Here's how the part is built. I have some questions about the finished solid (model axes, mm). Coordinates: 2 decimals unless noted, no trailing zeros. Write each loop counter-clockwise with the first axis right and the second up, starting at its lowest first coordinate (ties: lowest second). Pieces come first, ordered by that corner, then holes. Notation, with made-up numbers: (89, 62.25) -> (109, 62.25) arc R14 ccw to (109, 69.25) -> close; hole circle Ø10 at (62.25, -13). An arc over 180 degrees is marked (long way). Put each result on its own line as item: value. Start each with the question number.
Item 1: I want a section at D-D, the plane x = -8.5. List the corners of the cut face in (y, z) for me.
Item 2: For pin 1 (2 mm diameter, centred on x = -27, z = 4, fed in from +Y); pin 2 (3 mm diameter, centred on x = -3.5, y = 3.5, fed in from +Z); pin 3 (1 mm diameter, centred on x = -24, z = 2, fed in from -Y), each with a flat end and sliding along its axis, tell me the tip position at first contact or that it passes through.
Item 3: I want a section at A-A, the plane z = 1.4. List the corners of the cut face in (x, y) for me.
Item 4: I want a section at B-B, the plane y = 19. List the corners of the cut face in (x, z) for me, then the cut area to 3 significant figures.
Item 5: I need wall thicknesses on line 1 (Y direction, x = -3.5, z = 1.5); line 2 (X direction, y = 3.75, z = 4.55); line 3 (Y direction, x = -1.5, z = 2). Which ranges of each line are inside material? Lowest first, please. Write a range as [from, to].
Item 6: If we mould it in two halves opening along X, with no side actions, what happens to faces 1 (the face through (-17, 11, 5)), 2 (the face through (-5.003, 11.33, 2.465)), 3 (the face through (-16.83, 2.84, 2.46))? For each: released by +X, released by -X, zero draft, split by the parting line, or undercut.
Item 7: I want a section at C-C, the plane x = -30.5. List the corners of the cut face in (y, z) for me, then the cut area to 3 significant figures.
from build123d import *

# Parameters (mm, degrees)
ESQUISSE1_W        = 34
ESQUISSE1_H        = 22.5
ESQUISSE1_R        = 1
BOSS_EXTRU_1_DEPTH = 5
CUT_EXTRUDE1_DEPTH = 10


with BuildPart() as part:
    # Esquisse1 → Boss.-Extru.1 (new body)
    with BuildSketch(Plane.XY):
        with Locations((-17, 11.25)):
            Rectangle(ESQUISSE1_W, ESQUISSE1_H)
        with Locations((-30.5, 19)):
            Circle(ESQUISSE1_R, mode=Mode.SUBTRACT)
        with Locations((-3.5, 19)):
            Circle(ESQUISSE1_R, mode=Mode.SUBTRACT)
        with Locations((-3.5, 3.5)):
            Circle(ESQUISSE1_R, mode=Mode.SUBTRACT)
        with Locations((-30.5, 3.5)):
            Circle(ESQUISSE1_R, mode=Mode.SUBTRACT)
    extrude(amount=BOSS_EXTRU_1_DEPTH)

    # Sketch1 → Cut-Extrude1 (cut)
    with BuildSketch(Plane(origin=(0, 0, 0), x_dir=(-1, 0, 0), z_dir=(0, 0, -1))):
        Polygon((35.959040793, 25.036749556), (37.525504355, -3.285522646), (-6.460348748, -5.71831602), (-8.02681231, 22.603956182), align=None)
        with BuildLine():
            ThreePointArc((31.940553528, 15.810202901), (33.696545455, 20.425516451), (29.089552239, 22.203222926))
            ThreePointArc((29.089552239, 22.203222926), (17, 19.659419434), (4.910447761, 22.203222926))
            ThreePointArc((4.910447761, 22.203222926), (0.303454545, 20.425516451), (2.059446472, 15.810202901))
            ThreePointArc((2.059446472, 15.810202901), (5.003675676, 11.25), (2.059446472, 6.689797099))
            ThreePointArc((2.059446472, 6.689797099), (0.303454545, 2.074483549), (4.910447761, 0.296777074))
            ThreePointArc((4.910447761, 0.296777074), (17, 2.840580566), (29.089552239, 0.296777074))
            ThreePointArc((29.089552239, 0.296777074), (33.696545455, 2.074483549), (31.940553528, 6.689797099))
            ThreePointArc((31.940553528, 6.689797099), (28.996324324, 11.25), (31.940553528, 15.810202901))
        make_face(mode=Mode.SUBTRACT)
    extrude(amount=-CUT_EXTRUDE1_DEPTH, mode=Mode.SUBTRACT)


solid = part.part
Calculated:
1. outline: (1.61, 0) -> (20.89, 0) -> (20.89, 5) -> (1.61, 5) -> close
2. pin 1: stops at y = 21.75
2. pin 2: stops at z = 5
2. pin 3: stops at y = 1.89
3. outline: (-31.94, 6.69) arc R3.5 ccw to (-29.09, 0.3) arc R30 cw to (-4.91, 0.3) arc R3.5 ccw to (-2.06, 6.69) arc R5 cw to (-2.06, 15.81) arc R3.5 ccw to (-4.91, 22.2) arc R30 cw to (-29.09, 22.2) arc R3.5 ccw to (-31.94, 15.81) arc R5 cw to start; hole circle Ø2 at (-30.5, 3.5); hole circle Ø2 at (-30.5, 19); hole circle Ø2 at (-3.5, 3.5); hole circle Ø2 at (-3.5, 19)
4. outline: (-34, 0) -> (-31.5, 0) -> (-31.5, 5) -> (-34, 5) -> close; (-29.5, 0) -> (-4.5, 0) -> (-4.5, 5) -> (-29.5, 5) -> close; (-2.5, 0) -> (0, 0) -> (0, 5) -> (-2.5, 5) -> close
4. area: 150 mm2
5. line 1: y = [0, 2.5], [4.5, 7.67], [14.83, 18], [20, 22.5]
5. line 2: x = [-33.99, -31.47], [-29.53, -4.47], [-2.53, -0.01]
5. line 3: y = [0.63, 6.37], [16.13, 21.87]
6. face 1: zero draft
6. face 2: released by +X
6. face 3: undercut
7. outline: (0, 0) -> (2.5, 0) -> (2.5, 5) -> (0, 5) -> close; (4.5, 0) -> (7.67, 0) -> (7.67, 5) -> (4.5, 5) -> close; (14.83, 0) -> (18, 0) -> (18, 5) -> (14.83, 5) -> close; (20, 0) -> (22.5, 0) -> (22.5, 5) -> (20, 5) -> close
7. area: 56.7 mm2
